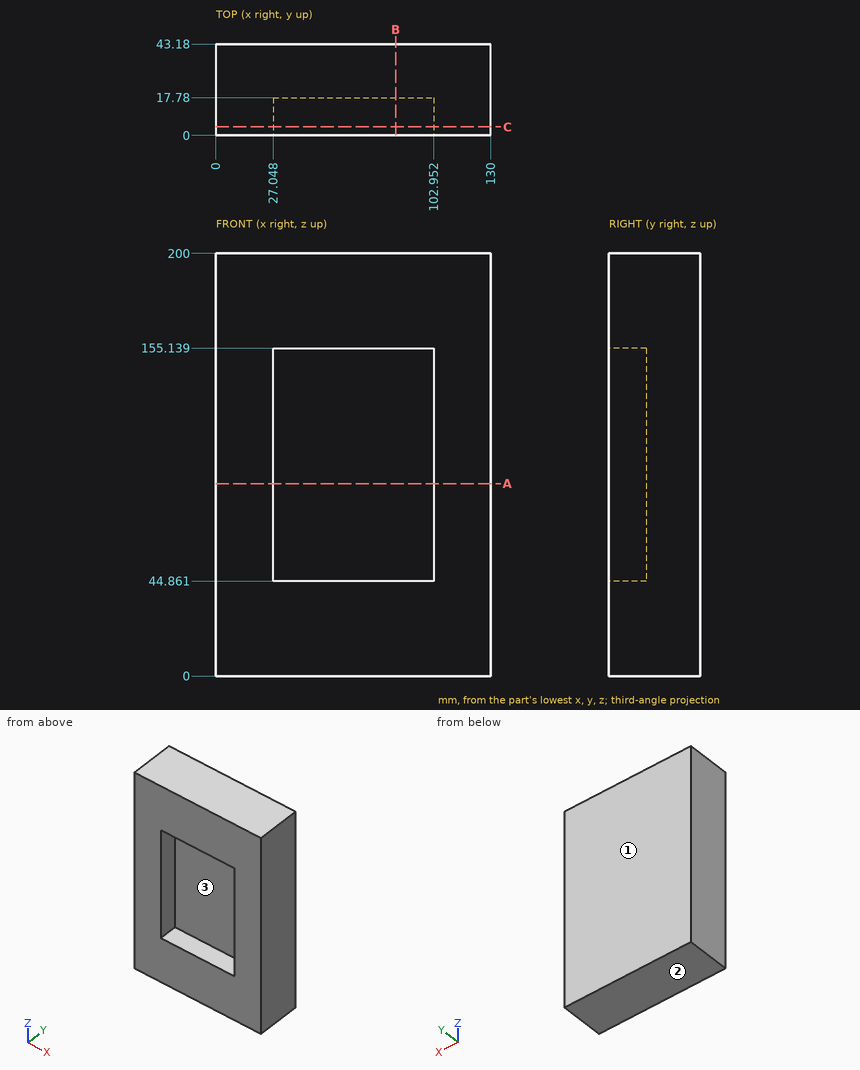
Can you work these out from the drawing? Everything is in mm from the part's minimum corner. Round coordinates to 2 decimals unless told otherwise and drop trailing zeros. Order: outer loops, then holes, each group sorted by start corner. A loop starts at its lowest first (then second) coordinate and runs counter-clockwise, first axis right, second up. Notation, with made-up numbers: (-16, 62) -> (19, 62) arc R27 ccw to (19, 101) -> close; hole circle Ø6 at (2.5, 51). An arc over 180 degrees is marked (long way). Return JSON: item names as keys, results as strings. Group by question number.
1. If we section it at C-C, the plane y = 4: Write out the boundary of the cut face in (x, z).
2. I need wall thicknesses on line 1 (Z direction, x = 39, y = 3); line 2 (X direction, y = 16, z = 75); line 3 (Y direction, x = 101.5, z = 61). Which ranges of each line are inside material? Lowest first, please. Write a range as [from, to].
3. We'd pull the mould along Z, two halves only. Please class the marked faces 1, 2 and 3: released by +Z, released by -Z, zero draft, split by the parting line, or undercut.
4. If we section it at A-A, the plane z = 91: Write out the boundary of the cut face in (x, y), then the cut area to 3 significant figures.
5. If we section it at B-B, the plane x = 85: Write out the boundary of the cut face in (y, z).
Output values:
{
 "1": {"outline": "(0, 0) -> (130, 0) -> (130, 200) -> (0, 200) -> close; hole (27.05, 44.86) -> (102.95, 44.86) -> (102.95, 155.14) -> (27.05, 155.14) -> close"},
 "2": {"line 1": "[0, 44.86], [155.14, 200]", "line 2": "[0, 27.05], [102.95, 130]", "line 3": "[17.78, 43.18]"},
 "3": {"face 1": "zero draft", "face 2": "released by -Z", "face 3": "undercut"},
 "4": {"outline": "(0, 0) -> (27.05, 0) -> (27.05, 17.78) -> (102.95, 17.78) -> (102.95, 0) -> (130, 0) -> (130, 43.18) -> (0, 43.18) -> close", "area": "4,260 mm²"},
 "5": {"outline": "(0, 0) -> (43.18, 0) -> (43.18, 200) -> (0, 200) -> (0, 155.14) -> (17.78, 155.14) -> (17.78, 44.86) -> (0, 44.86) -> close"}
}
